Here's the drawing with two shaded views (mm, measured from the low corner). I have some questions. Round coordinates to 2 decimals unless told otherwise and drop trailing zeros. Write each loop counter-clockwise with the first axis right and the second up, starting at its lowest first coordinate (ties: lowest second). Pieces come first, ordered by that corner, then holes. Notation, with made-up numbers: (76, 69.25) -> (100, 69.25) arc R12 cw to (100, 77.25) -> close; hole circle Ø10 at (20.25, 66.5). An arc over 180 degrees is marked (long way). Use CSV: the item, a comma, the result in double quotes.
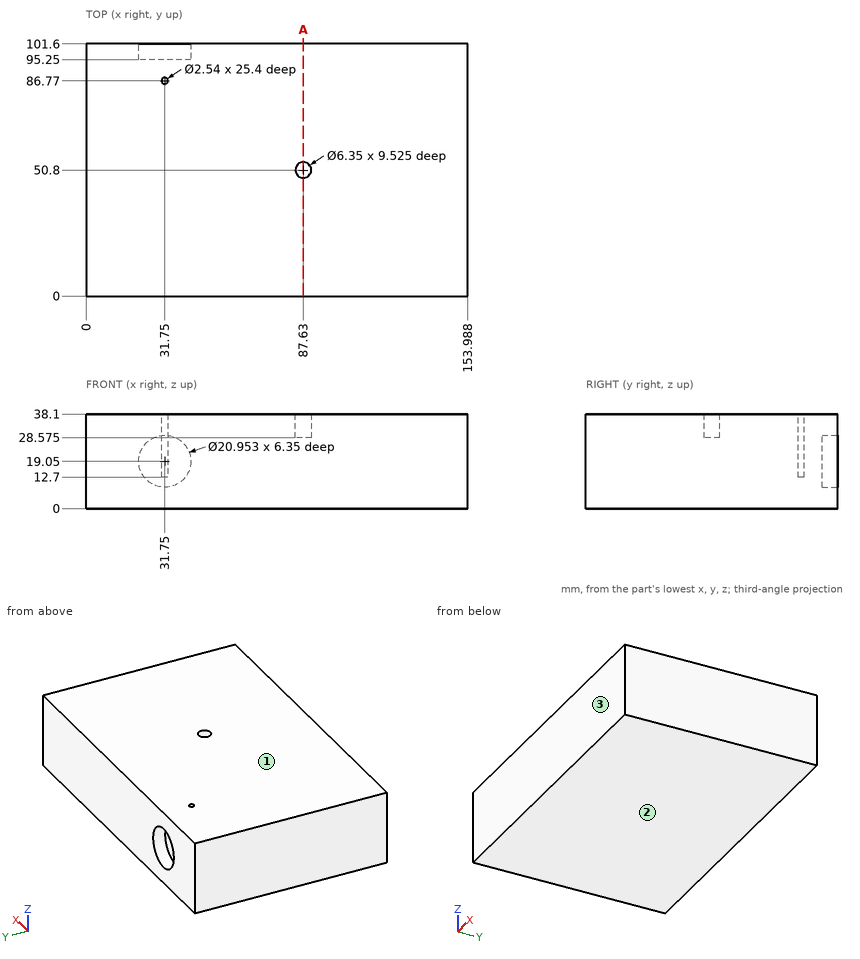
Q1. Will these pins go through, and if not, where does the flat tip stop? P1, Ø19, axis at x = 31.75, z = 19.05, coming from the +Y side; P2, Ø1.9, axis at x = 88, y = 51.5, coming from the +Z side (1 decimal); P3, Ø1.3, axis at x = 31.5, y = 87, coming from the +Z side.
Resolved:
P1,"stops at y = 95.25"
P2,"stops at z = 28.6"
P3,"stops at z = 12.7"
Q2. Suppose I cut it at A-A (x = 87.63). Write out the boundary of the cut face in (y, z) (1 decimal), and give its area (3 significant figures).
Resolved:
outline,"(0, 0) -> (101.6, 0) -> (101.6, 38.1) -> (54, 38.1) -> (54, 28.6) -> (47.6, 28.6) -> (47.6, 38.1) -> (0, 38.1) -> close"
area,"3,810 mm^2"
Q3. Please list where these lines run through material, in increasing order: probe 1 along X at (y, z) = (99.5, 19.05); probe 2 along X at (y, z) = (86, 18) (1 decimal); probe 3 along Y at (x, z) = (26, 13.5).
Resolved:
probe 1,"x = 0 to 21.27, 42.23 to 153.99"
probe 2,"x = 0 to 30.7, 32.8 to 154"
probe 3,"y = 0 to 95.25"
Q4. If we mould it in two halves opening along Z, with no side actions, what happens to the marked faces 1, 2 and 3? For each: released by +Z, released by -Z, zero draft, split by the parting line, or undercut.
Resolved:
face 1,"released by +Z"
face 2,"released by -Z"
face 3,"zero draft"
